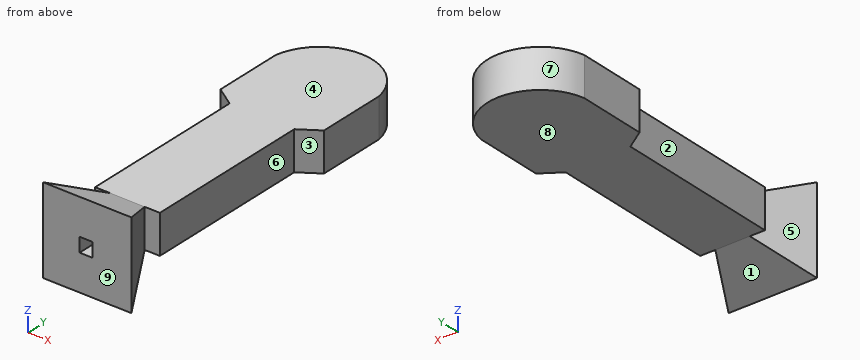
```python
from build123d import *

# Parameters (mm, degrees)
RESSALTO_EXTRUS_O2_DEPTH      = 4.5
RESSALTO_EXTRUS_O2_DEPTH_BACK = 4.5
CORTE_EXTRUS_O1_DEPTH         = 3.5
CORTE_EXTRUS_O1_DEPTH_BACK    = 3.5
RESSALTO_EXTRUS_O3_DEPTH      = 10.5
RESSALTO_EXTRUS_O3_DEPTH_BACK = 10
CORTE_EXTRUS_O2_DEPTH         = 20
CORTE_EXTRUS_O2_DEPTH_BACK    = 18.5
ESBO_O6_W                     = 3.02122436
ESBO_O6_H                     = 3.325672956
CORTE_EXTRUS_O3_DEPTH         = 17
CORTE_EXTRUS_O3_DEPTH_BACK    = 12.5


with BuildPart() as part:
    # Esboço1 → Ressalto-extrusão2 (new body, two sides)
    with BuildSketch(Plane.XY) as ressalto_extrus_o2_sk:
        with BuildLine():
            Line((-12, 1), (-12, -15))
            Line((-12, -15), (-7.5, -18))
            Line((-7.5, -18), (-7.5, -57))
            Line((-7.5, -57), (-4, -57))
            Line((-4, -57), (-10, -69))
            Line((-10, -69), (10, -69))
            Line((10, -69), (4, -57))
            Line((4, -57), (7.5, -57))
            Line((7.5, -57), (7.5, -18))
            Line((7.5, -18), (12, -15))
            Line((12, -15), (12, 1))
            ThreePointArc((12, 1), (0, 10.990932971), (-12, 1))
        make_face()
    extrude(amount=RESSALTO_EXTRUS_O2_DEPTH)
    extrude(ressalto_extrus_o2_sk.sketch, amount=-RESSALTO_EXTRUS_O2_DEPTH_BACK)

    # Esboço2 → Corte-extrusão1 (cut, two sides)
    with BuildSketch(Plane.XY) as corte_extrus_o1_sk:
        with BuildLine():
            Line((-8.5, -68), (8.5, -68))
            Line((8.5, -68), (3, -57.063736363))
            Line((3, -57.063736363), (3, -56.109442195))
            Line((3, -56.109442195), (6.5, -56.109442195))
            Line((6.5, -56.109442195), (6.5, -17.135100905))
            Line((6.5, -17.135100905), (11, -14))
            Line((11, -14), (11, 0))
            ThreePointArc((11, 0), (0, 9.976174937), (-11, 0))
            Line((-11, 0), (-11, -14))
            Line((-11, -14), (-6.5, -17.135100905))
            Line((-6.5, -17.135100905), (-6.5, -56.109442195))
            Line((-6.5, -56.109442195), (-3, -56.109442195))
            Line((-3, -56.109442195), (-3, -57.063736363))
            Line((-3, -57.063736363), (-8.5, -68))
        make_face()
    extrude(amount=CORTE_EXTRUS_O1_DEPTH, mode=Mode.SUBTRACT)
    extrude(corte_extrus_o1_sk.sketch, amount=-CORTE_EXTRUS_O1_DEPTH_BACK, mode=Mode.SUBTRACT)

    # Esboço4 → Ressalto-extrusão3 (add, two sides)
    with BuildSketch(Plane(origin=(0, 0, 0), x_dir=(0, 0, -1), z_dir=(1, 0, 0))) as ressalto_extrus_o3_sk:
        Polygon((0, -69), (10, -69), (4.5, -57), (-4.5, -57), (-10, -69), align=None)
    extrude(amount=RESSALTO_EXTRUS_O3_DEPTH)
    extrude(ressalto_extrus_o3_sk.sketch, amount=-RESSALTO_EXTRUS_O3_DEPTH_BACK)

    # Esboço5 → Corte-extrusão2 (cut, two sides)
    with BuildSketch(Plane.XY) as corte_extrus_o2_sk:
        Polygon((-4.015865961, -57), (-10, -69), (-10, -57), align=None)
        Polygon((3.984134039, -57), (10.5, -69), (10.5, -57), align=None)
    extrude(amount=CORTE_EXTRUS_O2_DEPTH, mode=Mode.SUBTRACT)
    extrude(corte_extrus_o2_sk.sketch, amount=-CORTE_EXTRUS_O2_DEPTH_BACK, mode=Mode.SUBTRACT)

    # Esboço6 → Corte-extrusão3 (cut, two sides)
    with BuildSketch(Plane(origin=(0, -69, 0), x_dir=(-1, 0, 0), z_dir=(0, -1, 0))) as corte_extrus_o3_sk:
        Rectangle(ESBO_O6_W, ESBO_O6_H)
    extrude(amount=CORTE_EXTRUS_O3_DEPTH, mode=Mode.SUBTRACT)
    extrude(corte_extrus_o3_sk.sketch, amount=-CORTE_EXTRUS_O3_DEPTH_BACK, mode=Mode.SUBTRACT)


solid = part.part
```
The model under review builds one solid part; all positions refer to its coordinate system, in mm. Face numbers are marked on the shaded views. A direction names the side the tool comes from. Round coordinates to 2 decimals unless told otherwise and drop trailing zeros. Write each loop counter-clockwise with the first axis right and the second up, starting at its lowest first coordinate (ties: lowest second). Pieces come first, ordered by that corner, then holes.
(1) Mouldability with a two-part tool opening along Y and no side actions: class the marked faces 1, 2, 3 and 4 as +Y half, -Y half, draft (parallel to the pull), parting line (faces both ways), or undercut.
(2) Insertion check: pin 1 (2 mm diameter, centred on y = -36.5, z = -0.5, fed in from -X); pin 2 (12 mm diameter, centred on x = -4.5, y = -17, fed in from +Z); pin 3 (4 mm diameter, centred on y = -52, z = -6, fed in from +X); pin 4 (10 mm diameter, centred on y = -16.5, z = -1.5, fed in from +X). Each pin has a flat end and moves straight along its axis. Give the tip position at first contact, or say it passes through.
(3) We need section C-C on z = -2.75. Give the boundary of the cut face in (x, y), and give its area (3 significant figures).
(4) Wall thickness on L1, parallel to X at y = -10.5, z = -2; L2, parallel to Y at x = 0.5, z = -2.25; L3, parallel to Y at x = -9.5, z = -2.25: over which ranges is each line inside the solid? List them lowest first.
(5) We need section A-A on x = 8.5. Give the boundary of the cut face in (y, z), and give its area (3 significant figures).
(6) We need section B-B on y = -20. Give the boundary of the cut face in (x, z), and give its area (3 significant figures).
(7) We need section D-D on y = -2. Give the boundary of the cut face in (x, z).
(8) Machinability: for the marked faces 5, 6, 7, 8 and 9, which of the approach directions +Z, -Z, +X, -X, +Y, -Y give a long, thin tool a straight path to every point of the face, cutting with its end or side? Answer none if there is none.
Findings below:
1. face 1: +Y half
1. face 2: undercut
1. face 3: undercut
1. face 4: draft
2. pin 1: stops at x = -7.5
2. pin 2: stops at z = 4.5
2. pin 3: stops at x = 7.5
2. pin 4: stops at x = 12
3. outline: (-12, -15) - (-7.5, -18) - (-7.5, -57) - (-4.02, -57) - (-10, -69) - (10.5, -69) - (3.98, -57) - (7.5, -57) - (7.5, -18) - (12, -15) - (12, 1) arc R12.2 ccw to (-12, 1) - close; hole (-11, -14) - (-6.5, -17.14) - (-6.5, -56.11) - (-3, -56.11) - (-3, -57) - (3, -57) - (3, -56.11) - (6.5, -56.11) - (6.5, -17.14) - (11, -14) - (11, 0) arc R11.05 ccw to (-11, 0) - close
3. area: 336 mm2
4. L1: x = -12 to -11, 11 to 12
4. L2: y = -69 to -57, 9.96 to 10.98
4. L3: y = -69 to -68, -16.67 to -15.05, 4.57 to 6.45
5. outline: (-69, -10) - (-65.32, -8.31) - (-65.32, 8.31) - (-69, 10) - close; (-17.33, -4.5) - (7.54, -4.5) - (7.54, 4.5) - (-17.33, 4.5) - close; hole (-15.74, -3.5) - (5.99, -3.5) - (5.99, 3.5) - (-15.74, 3.5) - close
5. area: 139 mm2
6. outline: (-7.5, -4.5) - (7.5, -4.5) - (7.5, 4.5) - (-7.5, 4.5) - close; hole (-6.5, -3.5) - (6.5, -3.5) - (6.5, 3.5) - (-6.5, 3.5) - close
6. area: 44.0 mm2
7. outline: (-12, -4.5) - (12, -4.5) - (12, 4.5) - (-12, 4.5) - close; hole (-11, -3.5) - (11, -3.5) - (11, 3.5) - (-11, 3.5) - close
8. face 5: +Z, -Z, -X
8. face 6: +Z, -Z, +X
8. face 7: +Z, -Z, +Y
8. face 8: -Z, +X, -X, +Y
8. face 9: +Z, -Z, +X, -X, -Y
